The model under review builds one solid part; all positions refer to its coordinate system, in mm. Face numbers are marked on the shaded views. A direction names the side the tool comes from. Give positions to 0.01 mm unless a question says otherwise; leave off trailing zeros. Loops run counter-clockwise (first coordinate to the right, second up) from the corner with the lowest first, then second, coordinate; pieces in that order, holes last. Notation, with made-up numbers: (52.25, 22) - (99.25, 22) arc R19 cw to (99.25, 58) - close; hole circle Ø5 at (49, 3). An arc over 180 degrees is marked (long way). Return JSON: item names as keys, results as strings. Group by question number.
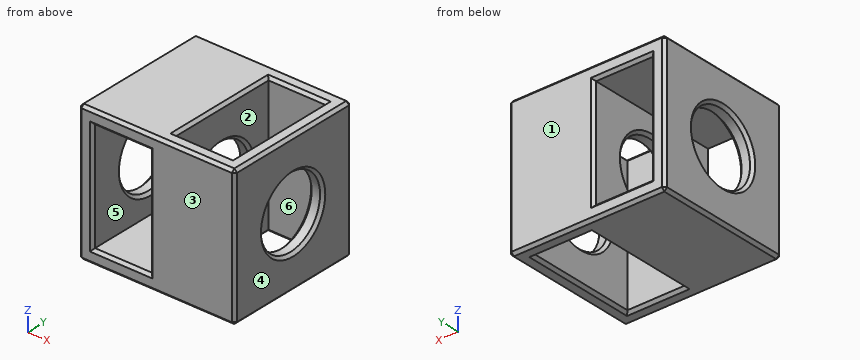
from build123d import *

# Parameters (mm, degrees)
SKETCH004_W          = 55.4
SKETCH004_H          = 49
PAD001_DEPTH         = 24.5
SKETCH005_W          = 20.2
SKETCH005_H          = 39
POCKET003_DEPTH      = 24.501
POCKET003_DEPTH_BACK = 24.501
SKETCH006_W          = 20.2
SKETCH006_H          = 39
POCKET004_DEPTH      = 24.501
POCKET004_DEPTH_BACK = 24.501
SKETCH007_R          = 12.5
POCKET005_DEPTH      = 27.701
POCKET005_DEPTH_BACK = 27.701
CHAMFER001_SIZE      = 1


with BuildPart() as part:
    # Sketch004 → Pad001 (new body, symmetric)
    with BuildSketch(Plane.XY):
        Rectangle(SKETCH004_W, SKETCH004_H)
    extrude(amount=PAD001_DEPTH, both=True)

    # Sketch005 → Pocket003 (cut, two sides)
    with BuildSketch(Plane.XY) as pocket003_sk:
        with Locations((12.6, 0)):
            Rectangle(SKETCH005_W, SKETCH005_H)
    extrude(amount=-POCKET003_DEPTH, mode=Mode.SUBTRACT)
    extrude(pocket003_sk.sketch, amount=POCKET003_DEPTH_BACK, mode=Mode.SUBTRACT)

    # Sketch006 → Pocket004 (cut, two sides)
    with BuildSketch(Plane.XZ) as pocket004_sk:
        with Locations((-12.6, 0)):
            Rectangle(SKETCH006_W, SKETCH006_H)
    extrude(amount=-POCKET004_DEPTH, mode=Mode.SUBTRACT)
    extrude(pocket004_sk.sketch, amount=POCKET004_DEPTH_BACK, mode=Mode.SUBTRACT)

    # Sketch007 → Pocket005 (cut, two sides)
    with BuildSketch(Plane.YZ) as pocket005_sk:
        Circle(SKETCH007_R)
    extrude(amount=-POCKET005_DEPTH, mode=Mode.SUBTRACT)
    extrude(pocket005_sk.sketch, amount=POCKET005_DEPTH_BACK, mode=Mode.SUBTRACT)

    # Chamfer001
    chamfer001_edges = [part.edges().sort_by_distance(p)[0] for p in [
        (-27.7, -24.5, 0),
        (0, -24.5, 24.5),
        (0, -24.5, -24.5),
        (27.7, -24.5, 0),
        (27.7, 0, 24.5),
        (-27.7, 0, 24.5),
        (0, 24.5, 24.5),
        (27.7, 24.5, 0),
        (27.7, 0, -24.5),
        (27.7, -12.5, 0),
        (22.7, -12.5, 0),
        (2.5, -12.5, 0),
        (2.5, 0, 24.5),
        (12.6, -19.5, 24.5),
        (22.7, 0, 24.5),
        (12.6, 19.5, 24.5),
        (-12.6, -24.5, 19.5),
        (-22.7, -24.5, 0),
        (-12.6, -24.5, -19.5),
        (-2.5, -24.5, 0),
        (-22.7, -12.5, 0),
        (-27.7, -12.5, 0),
        (-2.5, -12.5, 0),
        (0, 24.5, -24.5),
        (-27.7, 24.5, 0),
        (-22.7, 24.5, 0),
        (-2.5, 24.5, 0),
        (-12.6, 24.5, 19.5),
        (-12.6, 24.5, -19.5),
        (-27.7, 0, -24.5),
        (2.5, 0, -24.5),
        (12.6, -19.5, -24.5),
        (12.6, 19.5, -24.5),
        (22.7, 0, -24.5),
    ]]
    chamfer(chamfer001_edges, length=CHAMFER001_SIZE)


solid = part.part
Item 1: For L1, parallel to X at y = 8.5, z = 15.5; L2, parallel to Z at x = -5, y = 2; L3, parallel to Y at x = 25.7, z = 0, list the stretches that pass through material, from the lowest coordinate up. Write a range as from..to.
Item 2: Mouldability with a two-part tool opening along Y and no side actions: class the marked faces 1, 2 and 3 as +Y half, -Y half, draft (parallel to the pull), parting line (faces both ways), or undercut.
Item 3: Take a section at C-C (z = 0). State how many separate pieces and enclosed holes the cut face has, then the cut area to 3 significant figures.
Item 4: Tool access review of the marked faces 4, 5 and 6: name each direction out of +Z, -Z, +X, -X, +Y, -Y from which nothing blocks a thin tool from reaching the whole face with its end or side.
Item 5: Take a section at A-A (z = 15). State the section outline as (x, y) points.
Item 6: Take a section at B-B (x = 20). State the section outline as (y, z) points, then the cut area to 3 significant figures.
Item 7: For P1, Ø11.5, axis at y = 6.5, z = 3, coming from the +X side, flat-tipped, find the tip position at first contact; note if it passes through.
Check sheet entries:
{
 "1": {"L1": "x = -27.7..-22.7, -2.5..2.5, 22.7..27.7", "L2": "z = -24.5..-19.5, 19.5..24.5", "L3": "y = -24.5..-12.5, 12.5..24.5"},
 "2": {"face 1": "+Y half", "face 2": "undercut", "face 3": "-Y half"},
 "3": {"separate pieces": "4", "enclosed holes": "0", "area": "552 mm^2"},
 "4": {"face 4": "+Z, -Z, +X, +Y, -Y", "face 5": "+Y, -Y", "face 6": "+Z, -Z"},
 "5": {"outline": "(-27.7, -23.5) - (-26.7, -24.5) - (-23.7, -24.5) - (-22.7, -23.5) - (-22.7, 23.5) - (-23.7, 24.5) - (-26.7, 24.5) - (-27.7, 23.5) - close; (-2.5, -23.5) - (-1.5, -24.5) - (26.7, -24.5) - (27.7, -23.5) - (27.7, 23.5) - (26.7, 24.5) - (-1.5, 24.5) - (-2.5, 23.5) - close; hole (2.5, -19.5) - (22.7, -19.5) - (22.7, 19.5) - (2.5, 19.5) - close"},
 "6": {"outline": "(-24.5, -23.5) - (-23.5, -24.5) - (-20.5, -24.5) - (-19.5, -23.5) - (-19.5, 23.5) - (-20.5, 24.5) - (-23.5, 24.5) - (-24.5, 23.5) - close; (19.5, -23.5) - (20.5, -24.5) - (23.5, -24.5) - (24.5, -23.5) - (24.5, 23.5) - (23.5, 24.5) - (20.5, 24.5) - (19.5, 23.5) - close", "area": "486 mm^2"},
 "7": {"P1": "stops at x = 27.11"}
}
